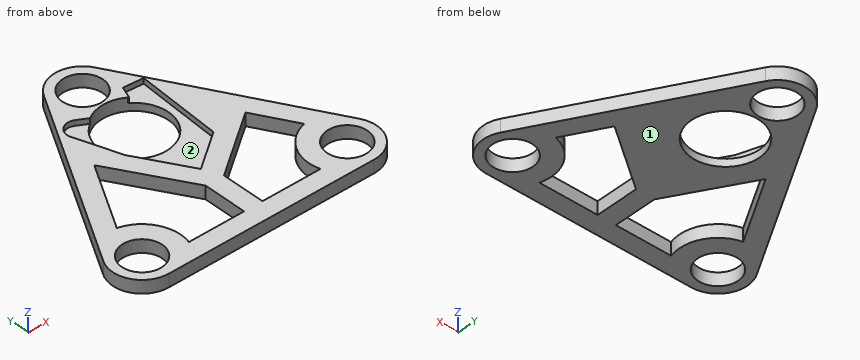
from build123d import *

# Parameters (mm, degrees)
SKETCH1_R           = 11
BOSS_EXTRUDE1_DEPTH = 7
SKETCH3_R           = 18.5
CUT_EXTRUDE1_DEPTH  = 8
CUT_EXTRUDE2_DEPTH  = 2.9
CUT_EXTRUDE3_DEPTH  = 8


with BuildPart() as part:
    # Sketch1 → Boss-Extrude1 (new body)
    with BuildSketch(Plane.XY):
        with BuildLine():
            Line((42.143593539, 104.994845224), (-13.856406461, 8))
            ThreePointArc((-13.856406461, 8), (-13.856406461, -8), (0, -16))
            Line((0, -16), (112, -16))
            ThreePointArc((112, -16), (125.856406461, -8), (125.856406461, 8))
            Line((125.856406461, 8), (69.856406461, 104.994845224))
            ThreePointArc((69.856406461, 104.994845224), (56, 112.994845224), (42.143593539, 104.994845224))
        make_face()
        Circle(SKETCH1_R, mode=Mode.SUBTRACT)
        with Locations((112, 0)):
            Circle(SKETCH1_R, mode=Mode.SUBTRACT)
        with Locations((56, 96.994845224)):
            Circle(SKETCH1_R, mode=Mode.SUBTRACT)
    extrude(amount=BOSS_EXTRUDE1_DEPTH)

    # Sketch3 → Cut-Extrude1 (cut, through all)
    with BuildSketch(Plane.XY.offset(7)):
        with Locations((56, 65.944845224)):
            Circle(SKETCH3_R)
    extrude(amount=-CUT_EXTRUDE1_DEPTH, mode=Mode.SUBTRACT)

    # Sketch4 → Cut-Extrude2 (cut)
    with BuildSketch(Plane.XY.offset(7)):
        with BuildLine():
            Line((46.11, 81.294845224), (66.94, 81.294845224))
            Line((66.94, 81.294845224), (69.163130932, 87.402847259))
            Line((69.163130932, 87.402847259), (79.735172855, 86.47791344))
            Line((79.735172855, 86.47791344), (76.482447168, 41.124405576))
            Line((76.482447168, 41.124405576), (56.230844768, 26.465872217))
            Line((56.230844768, 26.465872217), (39.901277947, 53.752961607))
            Line((39.901277947, 53.752961607), (31.804248297, 77.405405685))
            ThreePointArc((31.804248297, 77.405405685), (33.66849594, 83.981842037), (40.480834875, 84.544845224))
            Line((40.480834875, 84.544845224), (46.11, 81.294845224))
        make_face()
    extrude(amount=-CUT_EXTRUDE2_DEPTH, mode=Mode.SUBTRACT)

    # Sketch5 → Cut-Extrude3 (cut, through all)
    with BuildSketch(Plane.XY.offset(7)):
        with BuildLine():
            Line((26.139616059, 57.275143104), (4.866153476, 20.428425058))
            ThreePointArc((4.866153476, 20.428425058), (18.186533479, 10.5), (20.124611797, -6))
            Line((20.124611797, -6), (50.231546624, -6))
            Line((50.231546624, -6), (50.231546624, 17.016961725))
            Line((50.231546624, 17.016961725), (26.139616059, 57.275143104))
        make_face()
        with BuildLine():
            Line((60.231546624, 17.016961725), (60.231546624, -6))
            Line((60.231546624, -6), (91.875388203, -6))
            ThreePointArc((91.875388203, -6), (93.813466521, 10.5), (107.133846524, 20.428425058))
            Line((107.133846524, 20.428425058), (94.699401361, 41.965515845))
            Line((94.699401361, 41.965515845), (60.231546624, 17.016961725))
        make_face()
    extrude(amount=-CUT_EXTRUDE3_DEPTH, mode=Mode.SUBTRACT)


solid = part.part
CAD build for the part. Positions are in the model's coordinates, mm. Face numbers are marked on the shaded views. A direction names the side the tool comes from. Coordinates: 2 decimals unless noted, no trailing zeros. Write each loop counter-clockwise with the first axis right and the second up, starting at its lowest first coordinate (ties: lowest second). Pieces come first, ordered by that corner, then holes. Notation, with made-up numbers: M -4,88.25 L 9,88.25 A27 ccw 9,116.25 Z; hole C 69.25,7.25 d10. An arc over 180 degrees is marked long. Answer as a JSON object with one key per item and string values. Group by question number.
1) Saw through at D-D (x = 7). Write the cut outline in (y, z), plus the area to 3 significant figures.
2) Saw through at C-C (z = 5.25). Give the number of separate pieces and of enclosed holes in the cut face, plus the area to 4 significant figures.
3) Saw through at A-A (x = 118). Write the cut outline in (y, z).
4) Pin check, flat tips, straight feed: pin 1 Ø4 at (y, z) = (21, 4) entering from +X; pin 2 Ø1 at (y, z) = (44.5, 4.5) entering from +X; pin 3 Ø4 at (x, z) = (39, 3) entering from +Y. Stop position of each tip, or through.
5) Saw through at B-B (y = 92.5). Write the cut outline in (x, z).
6) Wall check: line 1 (Y direction, x = 56, z = 2.5); line 2 (X direction, y = 51.5, z = 4.75); line 3 (Y direction, x = 49, z = 2). Give the ranges that are in metal, low to high. Write a range as from..to.
7) Tool access for the marked faces 1 and 2: list every direction of +Z, -Z, +X, -X, +Y, -Y with a clear straight run to the whole face (end or side of a thin tool).
Values follow:
{
 "1": {"outline": "M -16,0 L -8.49,0 L -8.49,7 L -16,7 Z; M 8.49,0 L 19.8,0 L 19.8,7 L 8.49,7 Z; M 24.12,0 L 44.12,0 L 44.12,7 L 24.12,7 Z", "area": "272 mm2"},
 "2": {"separate pieces": "1", "enclosed holes": "6", "area": "5,505 mm2"},
 "3": {"outline": "M -14.83,0 L -9.22,0 L -9.22,7 L -14.83,7 Z; M 9.22,0 L 21.61,0 L 21.61,7 L 9.22,7 Z"},
 "4": {"pin 1": "stops at x = 119.51", "pin 2": "stops at x = 105.07", "pin 3": "stops at y = 103.01"},
 "5": {"outline": "M 34.93,0 L 45.96,0 L 45.96,7 L 34.93,7 Z; M 66.04,0 L 77.07,0 L 77.07,7 L 66.04,7 Z"},
 "6": {"line 1": "y = -16..47.44, 84.44..85.99, 107.99..112.99", "line 2": "x = 11.26..22.81, 29.6..41.25, 77.23..100.74", "line 3": "y = -16..-6, 19.07..48.82, 83.07..88.51, 105.48..111.38"},
 "7": {"face 1": "-Z, +X, -X, +Y, -Y", "face 2": "+Z"}
}
